Geometry check sheet. Reference: the model listing, model coordinates, mm. A direction names the side the tool comes from. Round coordinates to 2 decimals unless told otherwise and drop trailing zeros. Write each loop counter-clockwise with the first axis right and the second up, starting at its lowest first coordinate (ties: lowest second). Pieces come first, ordered by that corner, then holes. Notation, with made-up numbers: (25.25, 73.5) - (75.25, 73.5) arc R27 cw to (75.25, 110.5) - close; hole circle Ø11 at (-1.75, 48). An arc over 180 degrees is marked (long way). Return JSON: item names as keys, results as strings.
```python
from build123d import *

# Parameters (mm, degrees)
GRUNDPLATTE_DEPTH               = 4
SKIZZE2_R                       = 2
SCHNITT_LINEAR_AUSTRAGEN1_DEPTH = 83.559069762


with BuildPart() as part:
    # Skizze1 → Grundplatte (new body)
    with BuildSketch(Plane.XY):
        Polygon((80, 0), (-80, 0), (-80, -20), (-58, -20), (-51.287202951, -12), (51.287202951, -12), (58, -20), (80, -20), align=None)
    extrude(amount=GRUNDPLATTE_DEPTH)

    # Skizze2 → Schnitt-Linear austragen1 (cut, through all)
    with BuildSketch(Plane.XY.offset(4)):
        with Locations((-74, -10)):
            Circle(SKIZZE2_R)
        with Locations(Location((74, -10, 0), (0, 0, 180))):
            Circle(SKIZZE2_R)
    extrude(amount=-SCHNITT_LINEAR_AUSTRAGEN1_DEPTH, mode=Mode.SUBTRACT)


solid = part.part
```
(1) Material ranges on line 1 along Y through (x, z) = (-74, 2.25); line 2 along X through (y, z) = (-11.5, 2.65); line 3 along Y through (x, z) = (11, 0.7), recorded low to high. Write a range as [from, to].
Response values:
{"line 1": "y = [-20, -12], [-8, 0]", "line 2": "x = [-80, -75.32], [-72.68, 72.68], [75.32, 80]", "line 3": "y = [-12, 0]"}
(2) Gauge pin test, flat end, axial feed: pin 1 (2 mm diameter, centred on x = 14, z = 2.5, fed in from -Y). Record the tip position at first contact, or that the pin passes through.
Response values:
{"pin 1": "stops at y = -12"}
(3) Section check A-A, the plane y = -10. Enter the section's corners in (x, z), plus the area to 3 significant figures.
Response values:
{"outline": "(-80, 0) - (-76, 0) - (-76, 4) - (-80, 4) - close; (-72, 0) - (72, 0) - (72, 4) - (-72, 4) - close; (76, 0) - (80, 0) - (80, 4) - (76, 4) - close", "area": "608 mm^2"}
(4) Access from +Z, -Z, +X, -X, +Y, -Y to the whole of each face (thin tool, end or side, straight path). Record for faces 1 (the face through (1, 0, 2)), 2 (the face through (-54.691, -16.056, 1.972)).
Response values:
{"face 1": "+Z, -Z, +X, -X, +Y", "face 2": "+Z, -Z, -Y"}
(5) Section check B-B, the plane x = -74. Enter the section's corners in (y, z).
Response values:
{"outline": "(-20, 0) - (-12, 0) - (-12, 4) - (-20, 4) - close; (-8, 0) - (0, 0) - (0, 4) - (-8, 4) - close"}
(6) Section check D-D, the plane y = -17. Enter the section's corners in (x, z), plus the area to 3 significant figures.
Response values:
{"outline": "(-80, 0) - (-55.48, 0) - (-55.48, 4) - (-80, 4) - close; (55.48, 0) - (80, 0) - (80, 4) - (55.48, 4) - close", "area": "196 mm^2"}
(7) Section check C-C, the plane z = 1.45. Enter the section's corners in (x, y).
Response values:
{"outline": "(-80, -20) - (-58, -20) - (-51.29, -12) - (51.29, -12) - (58, -20) - (80, -20) - (80, 0) - (-80, 0) - close; hole circle Ø4 at (-74, -10); hole circle Ø4 at (74, -10)"}
